Study the drawing (mm; zero at the part's minimum x, y, z) and answer. Round coordinates to 2 decimals unless told otherwise and drop trailing zeros. Write each loop counter-clockwise with the first axis right and the second up, starting at its lowest first coordinate (ties: lowest second). Pieces come first, ordered by that corner, then holes.
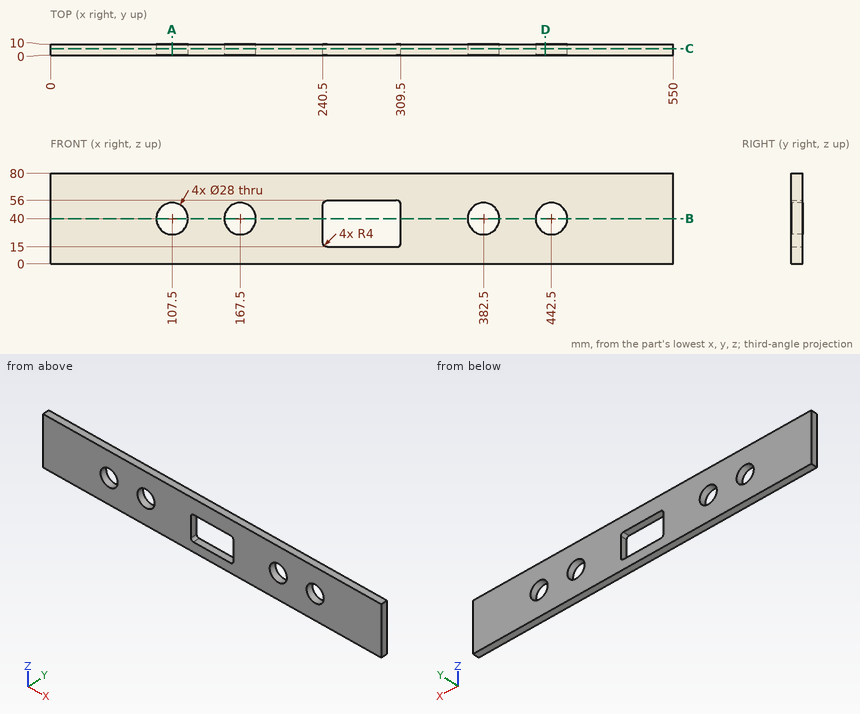
1. Section D-D on x = 437 is taken. Determine the outline of the cut face in (y, z).
Geometry says:
outline: (0, 0) - (10, 0) - (10, 27.13) - (0, 27.13) - close; (0, 52.87) - (10, 52.87) - (10, 80) - (0, 80) - close
2. Section C-C on y = 6 is taken. Determine the outline of the cut face in (x, z), plus the area to 3 significant figures.
Geometry says:
outline: (0, 0) - (550, 0) - (550, 80) - (0, 80) - close; hole circle Ø28 at (107.5, 40); hole circle Ø28 at (167.5, 40); hole (240.5, 19) arc R4 ccw to (244.5, 15) - (305.5, 15) arc R4 ccw to (309.5, 19) - (309.5, 52) arc R4 ccw to (305.5, 56) - (244.5, 56) arc R4 ccw to (240.5, 52) - close; hole circle Ø28 at (382.5, 40); hole circle Ø28 at (442.5, 40)
area: 38,700 mm2
3. Straight lines are drawn through the part: line 1 along X through (y, z) = (4.75, 32); line 2 along Z through (x, y) = (107.5, 2.75); line 3 along X through (y, z) = (8, 46). For each, find the intervals that lie inside material, in ascending order.
Geometry says:
line 1: x = 0 to 96.01, 118.99 to 156.01, 178.99 to 240.5, 309.5 to 371.01, 393.99 to 431.01, 453.99 to 550
line 2: z = 0 to 26, 54 to 80
line 3: x = 0 to 94.85, 120.15 to 154.85, 180.15 to 240.5, 309.5 to 369.85, 395.15 to 429.85, 455.15 to 550
4. Section B-B on z = 40 is taken. Determine the outline of the cut face in (x, y).
Geometry says:
outline: (0, 0) - (93.5, 0) - (93.5, 10) - (0, 10) - close; (121.5, 0) - (153.5, 0) - (153.5, 10) - (121.5, 10) - close; (181.5, 0) - (240.5, 0) - (240.5, 10) - (181.5, 10) - close; (309.5, 0) - (368.5, 0) - (368.5, 10) - (309.5, 10) - close; (396.5, 0) - (428.5, 0) - (428.5, 10) - (396.5, 10) - close; (456.5, 0) - (550, 0) - (550, 10) - (456.5, 10) - close
5. Section A-A on x = 107.5 is taken. Determine the outline of the cut face in (y, z).
Geometry says:
outline: (0, 0) - (10, 0) - (10, 26) - (0, 26) - close; (0, 54) - (10, 54) - (10, 80) - (0, 80) - close
